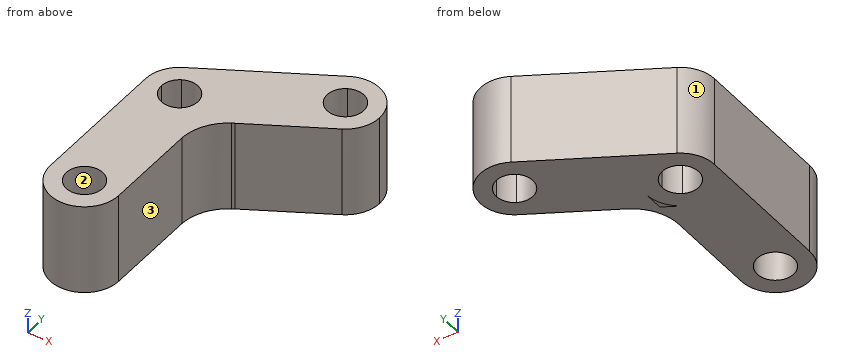
from build123d import *

# Parameters (mm, degrees)
F1_DEPTH = 12.7
F2_DEPTH = 12.7
F3_DEPTH = 12.7


with BuildPart() as f1:
    # F0 (on Top) → F1 (new body, symmetric)
    with BuildSketch(Plane.XY):
        with BuildLine():
            ThreePointArc((-16.7118934188, 0.0784563937), (-7.1868934188, -9.4465436063), (2.3381065812, 0.0784563937))
            Line((2.3381065812, 0.0784563937), (-2.1068934188, 0.0784563937))
            ThreePointArc((-2.1068934188, 0.0784563937), (-7.1868934188, -5.0015436063), (-12.2668934188, 0.0784563937))
            Line((-12.2668934188, 0.0784563937), (-16.7118934188, 0.0784563937))
        make_face()
        with BuildLine():
            ThreePointArc((-16.7118934188, 0.0784563937), (-7.1868934188, 9.6034563937), (2.3381065812, 0.0784563937))
            Line((2.3381065812, 0.0784563937), (2.3381065812, 24.6140933614))
            ThreePointArc((2.3381065812, 24.6140933614), (2.3310444619, 25.0462748775), (2.3381065812, 25.4784563937))
            Line((2.3381065812, 25.4784563937), (2.3381065812, 32.6791950797))
            Line((2.3381065812, 32.6791950797), (-2.4243934188, 29.9295644226))
            ThreePointArc((-2.4243934188, 29.9295644226), (-11.9493934188, 29.9295644226), (-16.7118934188, 38.1784563937))
            Line((-16.7118934188, 38.1784563937), (-16.7118934188, 0.0784563937))
        make_face()
        with BuildLine():
            Line((-2.1068934188, 0.0784563937), (2.3381065812, 0.0784563937))
            ThreePointArc((2.3381065812, 0.0784563937), (-7.1868934188, 9.6034563937), (-16.7118934188, 0.0784563937))
            Line((-16.7118934188, 0.0784563937), (-12.2668934188, 0.0784563937))
            ThreePointArc((-12.2668934188, 0.0784563937), (-7.1868934188, 5.1584563937), (-2.1068934188, 0.0784563937))
        make_face()
        with BuildLine():
            ThreePointArc((2.3381065812, 25.4784563937), (2.3310444619, 25.0462748775), (2.3381065812, 24.6140933614))
            Line((2.3381065812, 24.6140933614), (2.3381065812, 25.4784563937))
        make_face()
        with BuildLine():
            Line((2.3381065812, 32.6791950797), (2.3381065812, 25.4784563937))
            ThreePointArc((2.3381065812, 25.4784563937), (4.1032159035, 31.6601087373), (8.5741292093, 36.2795644226))
            Line((8.5741292093, 36.2795644226), (2.3381065812, 32.6791950797))
        make_face()
        with BuildLine():
            ThreePointArc((-11.9493934188, 46.4273483647), (-15.4357853898, 42.9409563937), (-16.7118934188, 38.1784563937))
            Line((-16.7118934188, 38.1784563937), (-12.2668934188, 38.1784563937))
            ThreePointArc((-12.2668934188, 38.1784563937), (-11.58630247, 40.7184563937), (-9.7268934188, 42.5778654449))
            Line((-9.7268934188, 42.5778654449), (-11.9493934188, 46.4273483647))
        make_face()
        with BuildLine():
            Line((-12.2668934188, 38.1784563937), (-16.7118934188, 38.1784563937))
            ThreePointArc((-16.7118934188, 38.1784563937), (-11.9493934188, 29.9295644226), (-2.4243934188, 29.9295644226))
            Line((-2.4243934188, 29.9295644226), (-4.6468934188, 33.7790473425))
            ThreePointArc((-4.6468934188, 33.7790473425), (-9.7268934188, 33.7790473425), (-12.2668934188, 38.1784563937))
        make_face()
        with BuildLine():
            Line((2.3381065812, 38.1784563937), (2.3381065812, 32.6791950797))
            Line((2.3381065812, 32.6791950797), (8.5741292093, 36.2795644226))
            ThreePointArc((8.5741292093, 36.2795644226), (8.9448783217, 36.5017711555), (9.3226895534, 36.7117459388))
            Line((9.3226895534, 36.7117459388), (30.5711744654, 48.9795644226))
            ThreePointArc((30.5711744654, 48.9795644226), (17.5597824944, 52.4659563937), (21.0461744654, 65.4773483647))
            Line((21.0461744654, 65.4773483647), (-11.9493934188, 46.4273483647))
            ThreePointArc((-11.9493934188, 46.4273483647), (-2.4243934188, 46.4273483647), (2.3381065812, 38.1784563937))
        make_face()
        with BuildLine():
            ThreePointArc((9.3226895534, 36.7117459388), (8.9448783217, 36.5017711555), (8.5741292093, 36.2795644226))
            Line((8.5741292093, 36.2795644226), (9.3226895534, 36.7117459388))
        make_face()
        with BuildLine():
            ThreePointArc((2.3381065812, 38.1784563937), (-2.4243934188, 46.4273483647), (-11.9493934188, 46.4273483647))
            Line((-11.9493934188, 46.4273483647), (-9.7268934188, 42.5778654449))
            ThreePointArc((-9.7268934188, 42.5778654449), (-4.6468934188, 42.5778654449), (-2.1068934188, 38.1784563937))
            Line((-2.1068934188, 38.1784563937), (2.3381065812, 38.1784563937))
        make_face()
        with BuildLine():
            ThreePointArc((35.3336744654, 57.2284563937), (30.5711744654, 65.4773483647), (21.0461744654, 65.4773483647))
            Line((21.0461744654, 65.4773483647), (23.2625173508, 61.6385298803))
            ThreePointArc((23.2625173508, 61.6385298803), (28.3548315801, 61.6385298803), (30.9009886947, 57.2284563937))
            ThreePointArc((30.9009886947, 57.2284563937), (30.218747952, 54.6822992791), (28.3548315801, 52.8183829071))
            Line((28.3548315801, 52.8183829071), (30.5711744654, 48.9795644226))
            ThreePointArc((30.5711744654, 48.9795644226), (34.0575664365, 52.4659563937), (35.3336744654, 57.2284563937))
        make_face()
        with BuildLine():
            Line((23.2625173508, 61.6385298803), (21.0461744654, 65.4773483647))
            ThreePointArc((21.0461744654, 65.4773483647), (17.5597824944, 52.4659563937), (30.5711744654, 48.9795644226))
            Line((30.5711744654, 48.9795644226), (28.3548315801, 52.8183829071))
            ThreePointArc((28.3548315801, 52.8183829071), (21.3986009788, 54.6822992791), (23.2625173508, 61.6385298803))
        make_face()
    extrude(amount=F1_DEPTH, both=True)

    # F0 (on Top) → F2 (join, symmetric)
    with BuildSketch(Plane.XY):
        with BuildLine():
            Line((-4.6468934188, 33.7790473425), (-2.4243934188, 29.9295644226))
            ThreePointArc((-2.4243934188, 29.9295644226), (1.0619985523, 33.4159563937), (2.3381065812, 38.1784563937))
            Line((2.3381065812, 38.1784563937), (-2.1068934188, 38.1784563937))
            ThreePointArc((-2.1068934188, 38.1784563937), (-2.7874843675, 35.6384563937), (-4.6468934188, 33.7790473425))
        make_face()
    extrude(amount=F2_DEPTH, both=True)

    # F0 (on Top) → F3 (join, symmetric)
    with BuildSketch(Plane.XY):
        with BuildLine():
            Line((-2.4243934188, 29.9295644226), (2.3381065812, 32.6791950797))
            Line((2.3381065812, 32.6791950797), (2.3381065812, 38.1784563937))
            ThreePointArc((2.3381065812, 38.1784563937), (1.0619985523, 33.4159563937), (-2.4243934188, 29.9295644226))
        make_face()
    extrude(amount=F3_DEPTH, both=True)


solid = f1.part
The model under review builds one solid part; all positions refer to its coordinate system, in mm. Face numbers are marked on the shaded views. Round coordinates to 2 decimals unless told otherwise and drop trailing zeros. Write each loop counter-clockwise with the first axis right and the second up, starting at its lowest first coordinate (ties: lowest second). Pieces come first, ordered by that corner, then holes. Notation, with made-up numbers: (30, -32.5) -> (67, -32.5) arc R14 ccw to (67, -6.5) -> close; hole circle Ø7 at (-23, 57.5). An arc over 180 degrees is marked (long way). Answer as a JSON object with one key per item and string values.
1. We need section A-A on z = 10. State the section outline as (x, y) points (3 decimals), and give its area (3 significant figures).
Results found:
{"outline": "(-16.712, 0.078) arc R9.525 ccw to (2.338, 0.078) -> (2.338, 25.478) arc R13.228 cw to (8.574, 36.28) -> (30.571, 48.98) arc R9.525 ccw to (21.046, 65.477) -> (-11.949, 46.427) arc R9.525 ccw to (-16.712, 38.178) -> close; hole circle Ø10.16 at (-7.187, 0.078); hole circle Ø10.16 at (-7.187, 38.178); hole circle Ø10.185 at (25.809, 57.228)", "area": "1,500 mm^2"}
2. We need section C-C on y = 59. State the section outline as (x, z) points.
Results found:
{"outline": "(9.83, -12.7) -> (21.03, -12.7) -> (21.03, 12.7) -> (9.83, 12.7) -> close; (30.58, -12.7) -> (35.17, -12.7) -> (35.17, 12.7) -> (30.58, 12.7) -> close"}
3. To check wall thickness, follow line 1 along Y through (x, z) = (-11.5, -10); line 2 along X through (y, z) = (0, -9); line 3 along Y through (x, z) = (-5, -10.5). State the ranges of each line that lie inside material, in increasing order.
Results found:
{"line 1": "y = -8.41 to -2.61, 2.76 to 35.49, 40.86 to 46.69", "line 2": "x = -16.71 to -12.27, -2.11 to 2.34", "line 3": "y = -9.19 to -4.51, 4.66 to 33.59, 42.76 to 50.44"}
4. We need section B-B on x = 26. State the section outline as (y, z) points, and give its area (3 significant figures).
Results found:
{"outline": "(46.34, -12.7) -> (52.14, -12.7) -> (52.14, 12.7) -> (46.34, 12.7) -> close; (62.32, -12.7) -> (66.75, -12.7) -> (66.75, 12.7) -> (62.32, 12.7) -> close", "area": "260 mm^2"}
5. The part is to be moulded in two halves that separate along Y. For the marked faces 1, 2 and 3, say which applies: pulls with the +Y half, pulls with the -Y half, needs draft (parallel to the pull), parting line crosses it, or undercut.
Results found:
{"face 1": "pulls with the +Y half", "face 2": "undercut", "face 3": "needs draft"}
6. Clearance check with flat-ended pins moving along their axes: pin 1 (4 mm diameter, centred on x = 0, z = 1, fed in from +Y); pin 2 (6 mm diameter, centred on y = 29.5, z = -6.5, fed in from +X); pin 3 (5 mm diameter, centred on x = -11.5, z = 4.5, fed in from +Y); pin 4 (8 mm diameter, centred on x = -7.19, y = 0.08, fed in from -Z). State where each tip first meets the part, or that it passes through.
Results found:
{"pin 1": "stops at y = 54.48", "pin 2": "stops at x = 4.63", "pin 3": "stops at y = 48.13", "pin 4": "passes through"}
7. We need section D-D on y = 12. State the section outline as (x, z) points, and give its area (3 significant figures).
Results found:
{"outline": "(-16.71, -12.7) -> (2.34, -12.7) -> (2.34, 12.7) -> (-16.71, 12.7) -> close", "area": "484 mm^2"}
